Geometry: see drawing. Coordinates: mm, zero at the bounding-box minimum. Give positions to 0.01 mm unless a question says otherwise; leave off trailing zeros. Loops run counter-clockwise (first coordinate to the right, second up) from the corner with the lowest first, then second, coordinate; pieces in that order, holes last. Notation, with made-up numbers: M 63,-7 L 95,-7 A9 cw 95,-2 Z; hole C -34,53 d9. An arc over 180 degrees is marked long. Use a Markdown table: item, result. Add a question column.
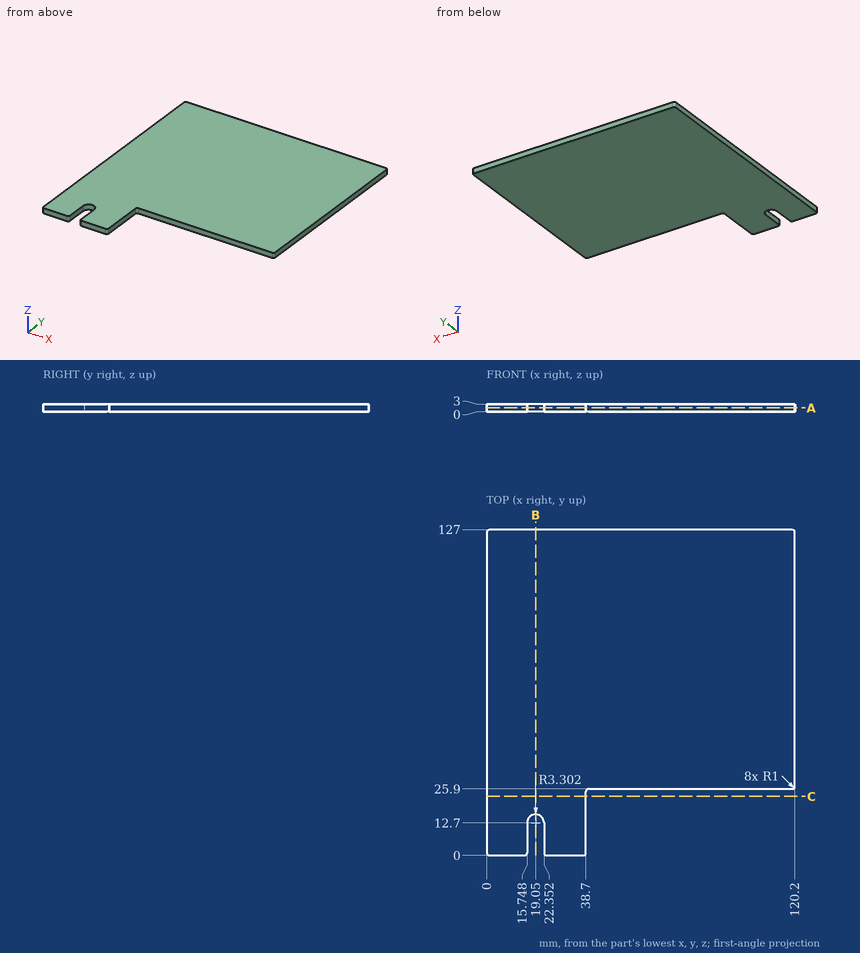
1) Section query C-C, the plane y = 23. Return the cut outline in (x, z).
2) Section query B-B, the plane x = 19.05. Return the cut outline in (y, z).
3) Ray query, line 1 (Y direction, x = 103, z = 0.35). Return the intervals inside material, ascending. Write a range as [from, to].
4) Contact query for flat-ended pins moving along their axis: P1, Ø1, axis at y = 20, z = 1, coming from the +X side; P2, Ø0.9, axis at x = 80.5, z = 1.5, coming from the -Y side. Output: stop coordinate, or through.
5) Section query A-A, the plane z = 1.45. Return the cut outline in (x, y).
Entries:
| question | item | result |
|---|---|---|
| 1 | outline | M 0,0 L 38.7,0 L 38.7,3 L 0,3 Z |
| 2 | outline | M 16,0 L 127,0 L 127,3 L 16,3 Z |
| 3 | line 1 | y = [25.9, 127] |
| 4 | P1 | stops at x = 38.7 |
| 4 | P2 | stops at y = 25.9 |
| 5 | outline | M 0,1 A1 ccw 1,0 L 14.75,0 A1 ccw 15.75,1 L 15.75,12.7 A3.3 cw 22.35,12.7 L 22.35,1 A1 ccw 23.35,0 L 37.7,0 A1 ccw 38.7,1 L 38.7,24.9 A1 cw 39.7,25.9 L 119.2,25.9 A1 ccw 120.2,26.9 L 120.2,126 A1 ccw 119.2,127 L 1,127 A1 ccw 0,126 Z |
